Build history of the part. All positions in model axes, mm. Face numbers are marked on the shaded views. A direction names the side the tool comes from. Give positions to 0.01 mm unless a question says otherwise; leave off trailing zeros. Order: outer loops, then holes, each group sorted by start corner. A loop starts at its lowest first (then second) coordinate and runs counter-clockwise, first axis right, second up. Notation, with made-up numbers: (-34, 38.5) - (-28, 38.5) arc R19 ccw to (-28, 66.5) - close; hole circle Ø1 at (-9, 11.25). An arc over 180 degrees is marked (long way). Write each question's results on one line, items separated by ' | '. Start each with the question number.
1) Drill centre lines: line 1 along X through (y, z) = (7.5, -23) (3 decimals); line 2 along Z through (x, y) = (28, 5); line 3 along Z through (x, y) = (43.5, -46.5). Where is each one in solid material? Low to high. Write a range as from..to.
2) Cut at C-C on y = -30.5. List the corners of the cut face in (x, z).
3) Cut at D-D on x = 40.5. List the corners of the cut face in (y, z), plus the area to 3 significant figures.
4) Cut at B-B on x = 30. List the corners of the cut face in (y, z).
5) Cut at A-A on z = -19. List the corners of the cut face in (x, y) (3 decimals), plus the area to 3 significant figures.
6) Tool access for the marked faces 1, 2, 3 and 4: list every direction of +Z, -Z, +X, -X, +Y, -Y with a clear straight run to the whole face (end or side of a thin tool).
7) Two-plate mould, pull along X, no slides. Class the marked faces 5, 6 and 7: +X half, -X half, draft (parallel to the pull), parting line (faces both ways), or undercut.
from build123d import *

# Parameters (mm, degrees)
SKETCH1_W               = 57.15
SKETCH1_H               = 33
BOSS_EXTRUDE1_DEPTH     = 10
SKETCH2_W               = 4.2
SKETCH2_H               = 11
CUT_EXTRUDE1_DEPTH      = 5.8
BOSS_EXTRUDE2_START     = -43.975
BOSS_EXTRUDE2_DEPTH     = 55.8
SKETCH4_W               = 33
SKETCH4_H               = 2.2
CUT_EXTRUDE2_DEPTH      = 1
CUT_EXTRUDE2_DEPTH_BACK = 58.15
FILLET1_R               = 2
SKETCH7_W               = 20.8
SKETCH7_H               = 17
CUT_EXTRUDE4_DEPTH      = 16
FILLET2_R               = 2
BOSS_EXTRUDE4_START     = -7.8
SKETCH5_W               = 57.15
SKETCH5_H               = 5
BOSS_EXTRUDE4_DEPTH     = 52.15
SKETCH8_W               = 47.15
SKETCH8_H               = 47.15
CUT_EXTRUDE5_DEPTH      = 52.15
FILLET3_R               = 10
FILLET4_R               = 5


with BuildPart() as part:
    # Sketch1 → Boss-Extrude1 (new body)
    with BuildSketch(Plane(origin=(0, 0, 0), x_dir=(1, 0, 0), z_dir=(0, 1, 0))):
        with Locations((28.575, 16.5)):
            Rectangle(SKETCH1_W, SKETCH1_H)
    extrude(amount=BOSS_EXTRUDE1_DEPTH)

    # Sketch2 → Cut-Extrude1 (cut)
    with BuildSketch(Plane(origin=(0, 10, 0), x_dir=(1, 0, 0), z_dir=(0, 1, 0))):
        with Locations((11.075, 23)):
            Rectangle(SKETCH2_W, SKETCH2_H)
        with Locations((46.075, 23)):
            Rectangle(SKETCH2_W, SKETCH2_H)
    extrude(amount=-CUT_EXTRUDE1_DEPTH, mode=Mode.SUBTRACT)

    # Sketch3 → Boss-Extrude2 (add)
    with BuildSketch(Plane.ZY.offset(-13.175).offset(BOSS_EXTRUDE2_START)):
        Polygon((-28.5, 5.85), (-25.1, 8.5), (-25.1, 10), (-28.5, 10), align=None)
    extrude(amount=BOSS_EXTRUDE2_DEPTH)

    # Sketch4 → Cut-Extrude2 (cut, two sides)
    with BuildSketch(Plane(origin=(57.15, 0, 0), x_dir=(0, 0, -1), z_dir=(1, 0, 0))) as cut_extrude2_sk:
        with Locations((16.5, 1.1)):
            Rectangle(SKETCH4_W, SKETCH4_H)
    extrude(amount=CUT_EXTRUDE2_DEPTH, mode=Mode.SUBTRACT)
    extrude(cut_extrude2_sk.sketch, amount=-CUT_EXTRUDE2_DEPTH_BACK, mode=Mode.SUBTRACT)

    # Fillet1
    fillet1_edges = [part.edges().sort_by_distance(p)[0] for p in [
        (11.075, 10, -17.5),
        (46.075, 10, -17.5),
    ]]
    fillet(fillet1_edges, radius=FILLET1_R)

    # Sketch7 → Cut-Extrude4 (cut)
    with BuildSketch(Plane(origin=(0, 10, 0), x_dir=(1, 0, 0), z_dir=(0, 1, 0))):
        with Locations((28.575, 19.5)):
            Rectangle(SKETCH7_W, SKETCH7_H)
    extrude(amount=-CUT_EXTRUDE4_DEPTH, mode=Mode.SUBTRACT)

    # Fillet2
    fillet2_edges = [part.edges().sort_by_distance(p)[0] for p in [
        (18.175, 6.1, -11),
        (18.175, 6.1, -28),
        (38.975, 6.1, -28),
        (38.975, 6.1, -11),
    ]]
    fillet(fillet2_edges, radius=FILLET2_R)

    # Sketch5 → Boss-Extrude4 (add)
    with BuildSketch(Plane(origin=(0, 10, 0), x_dir=(1, 0, 0), z_dir=(0, 1, 0)).offset(BOSS_EXTRUDE4_START)):
        with Locations((28.575, 2.5)):
            Rectangle(SKETCH5_W, SKETCH5_H)
    extrude(amount=-BOSS_EXTRUDE4_DEPTH)

    # Sketch8 → Cut-Extrude5 (cut)
    with BuildSketch(Plane(origin=(0, 0, -5), x_dir=(-1, 0, 0), z_dir=(0, 0, -1))):
        with Locations((-28.575, -21.375)):
            Rectangle(SKETCH8_W, SKETCH8_H)
    extrude(amount=-CUT_EXTRUDE5_DEPTH, mode=Mode.SUBTRACT)

    # Fillet3
    fillet3_edges = [part.edges().sort_by_distance(p)[0] for p in [
        (54.65, 2.2, -5),
        (2.5, 2.2, -5),
        (52.15, -44.95, -2.5),
        (52.15, 2.2, -2.5),
        (5, 2.2, -2.5),
        (5, -44.95, -2.5),
    ]]
    fillet(fillet3_edges, radius=FILLET3_R)

    # Fillet4
    fillet4_edges = [part.edges().sort_by_distance(p)[0] for p in [
        (57.15, -49.95, -2.5),
        (0, -49.95, -2.5),
    ]]
    fillet(fillet4_edges, radius=FILLET4_R)


solid = part.part
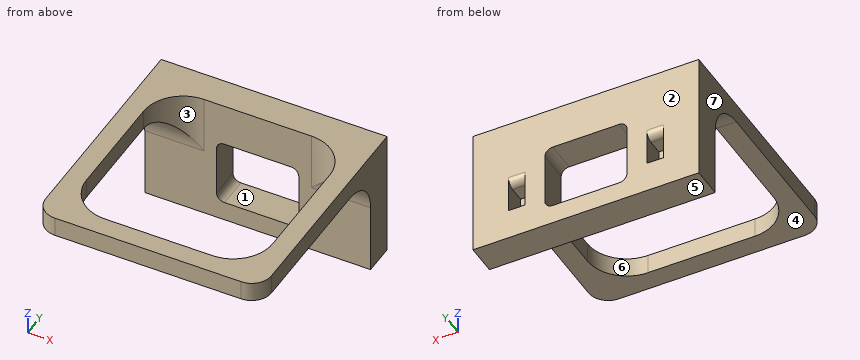
Results:
1) line 1: 0..8.975, 13.175..18.175, 38.975..43.975, 48.175..57.15 | line 2: -33..-28, -11..0 | line 3: -5..0
2) outline: (0, -5) - (5, -5) - (5, 0) - (0, 0) - close; (52.15, -5) - (57.15, -5) - (57.15, 0) - (52.15, 0) - close
3) outline: (-49.95, -5) - (-44.95, -5) - (-44.95, 0) - (-49.95, 0) - close; (2.2, -33) - (10, -33) - (10, 0) - (2.2, 0) - close | area: 282 mm^2
4) outline: (-49.95, -5) - (-44.95, -5) - (-44.95, 0) - (-49.95, 0) - close; (2.2, -33) - (10, -33) - (10, -28) - (2.2, -28) - close; (2.2, -11) - (10, -11) - (10, 0) - (2.2, 0) - close
5) outline: (0, 2.2) - (18.175, 2.2) - (18.175, 10) - (13.175, 10) - (13.175, 4.2) - (8.975, 4.2) - (8.975, 10) - (0, 10) - close; (38.975, 2.2) - (57.15, 2.2) - (57.15, 10) - (48.175, 10) - (48.175, 4.2) - (43.975, 4.2) - (43.975, 10) - (38.975, 10) - close | area: 235 mm^2
6) face 1: +Y, -Y | face 2: +Z, -Z, +X, -X, +Y | face 3: +Z, -Z | face 4: -Z, +X, -X, -Y
7) face 5: draft | face 6: undercut | face 7: -X half
